Build history of the part. All positions in model axes, mm. Face numbers are marked on the shaded views. A direction names the side the tool comes from. Give positions to 0.01 mm unless a question says otherwise; leave off trailing zeros. Write each loop counter-clockwise with the first axis right and the second up, starting at its lowest first coordinate (ties: lowest second). Pieces come first, ordered by that corner, then holes.
from build123d import *

# Parameters (mm, degrees)
F0_R     = 3
F1_DEPTH = 60
F2_R     = 5
F3_DEPTH = 4
F4_R     = 0.5
F5_W     = 13
F5_H     = 2
F6_DEPTH = 2.3


with BuildPart() as f1:
    # F0 (on Top) → F1 (new body)
    with BuildSketch(Plane.XY):
        Circle(F0_R)
    extrude(amount=-F1_DEPTH)

    # F2 (on face) → F3 (join)
    with BuildSketch(Plane.XY):
        Circle(F2_R)
    extrude(amount=F3_DEPTH)

    # F4
    f4_edges = [f1.edges().sort_by_distance(p)[0] for p in [
        (-5, 0, 4),
        (-5, 0, 0),
    ]]
    fillet(f4_edges, radius=F4_R)

    # F5 (on face) → F6 (cut)
    with BuildSketch(Plane.XY.offset(4)):
        Rectangle(F5_W, F5_H)
    extrude(amount=-F6_DEPTH, mode=Mode.SUBTRACT)


solid = f1.part
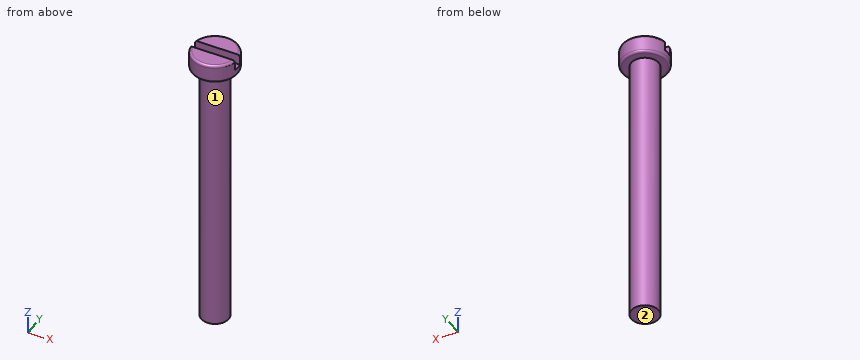
(1) 3-axis set-ups, long thin cutter, end or side, ignore diameter. For the marked faces 1 and 2: which of +Z, -Z, +X, -X, +Y, -Y reach the whole face in a straight line?
(2) Saw through at C-C, the plane z = -2. List the corners of the cut face in (x, y).
(3) Drop flat-ended pins along their axis: pin 1 (1.2 mm diameter, centred on x = 1.5, z = 2.5, fed in from +Y); pin 2 (5 mm diameter, centred on x = 1.5, z = -37.5, fed in from +Y); pin 3 (4 mm diameter, centred on x = 3.5, z = -20, fed in from +Y). Give the stop position or say it passes through.
(4) Saw through at B-B, the plane x = 0. List the corners of the cut face in (y, z), plus the area to 3 significant figures.
(5) Saw through at A-A, the plane y = 0. List the corners of the cut face in (x, z), plus the area to 3 significant figures.
(6) Probe line 1 (Z direction, x = 0.5, y = -3.25); line 2 (Z direction, x = 0, y = 0); line 3 (X direction, y = -1.5, z = -9). List the from-to ranges inside material, lowest first.
Computed values:
1. face 1: -Z
1. face 2: -Z, +X, -X, +Y, -Y
2. outline: circle Ø6 at (0, 0)
3. pin 1: stops at y = 4.92
3. pin 2: stops at y = 3
3. pin 3: stops at y = 2.6
4. outline: (-5, 0.5) arc R0.5 ccw to (-4.5, 0) - (-3, 0) - (-3, -60) - (3, -60) - (3, 0) - (4.5, 0) arc R0.5 ccw to (5, 0.5) - (5, 3.5) arc R0.5 ccw to (4.5, 4) - (1, 4) - (1, 1.7) - (-1, 1.7) - (-1, 4) - (-4.5, 4) arc R0.5 ccw to (-5, 3.5) - close
4. area: 395 mm2
5. outline: (-5, 0.5) arc R0.5 ccw to (-4.5, 0) - (-3, 0) - (-3, -60) - (3, -60) - (3, 0) - (4.5, 0) arc R0.5 ccw to (5, 0.5) - (5, 1.7) - (-5, 1.7) - close
5. area: 377 mm2
6. line 1: z = 0 to 4
6. line 2: z = -60 to 1.7
6. line 3: x = -2.6 to 2.6
